Check sheet for the drawn part. Datum: minimum x, y, z corner. Units: mm. Give positions to 0.01 mm unless a question says otherwise; leave off trailing zeros. Order: outer loops, then holes, each group sorted by start corner. A loop starts at its lowest first (then second) coordinate and runs counter-clockwise, first axis right, second up.
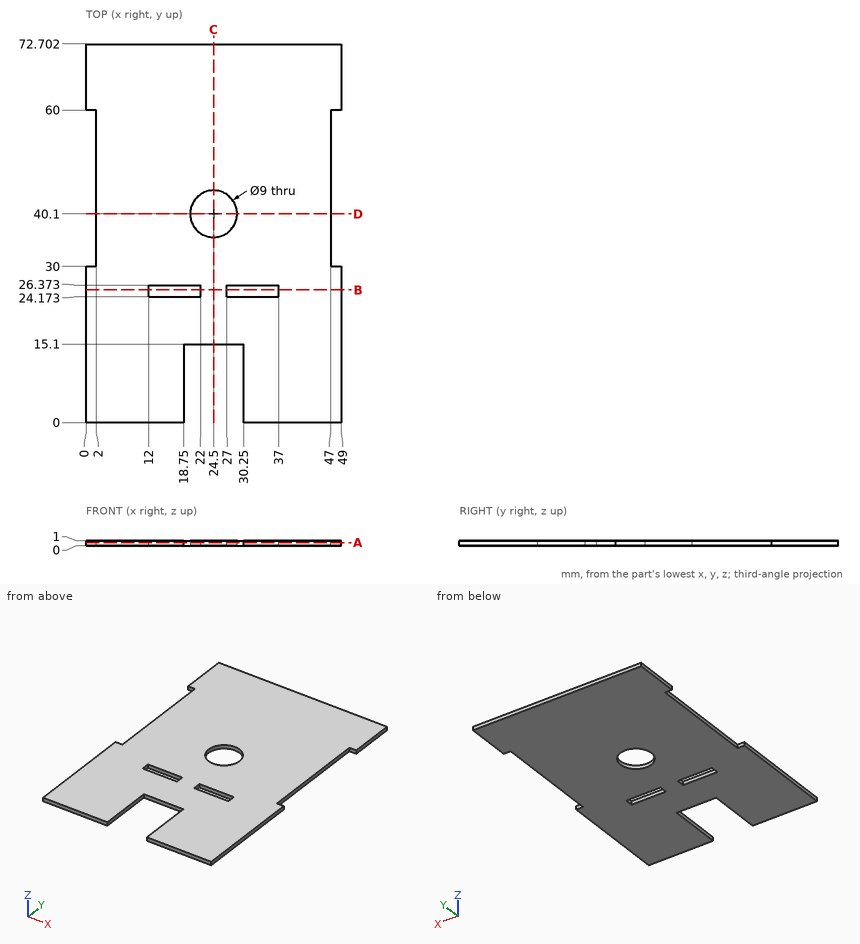
(1) Section check A-A, the plane z = 0.65. Enter the section's corners in (x, y).
Solved:
outline: (0, 0) - (18.75, 0) - (18.75, 15.1) - (30.25, 15.1) - (30.25, 0) - (49, 0) - (49, 30) - (47, 30) - (47, 60) - (49, 60) - (49, 72.7) - (0, 72.7) - (0, 60) - (2, 60) - (2, 30) - (0, 30) - close; hole (12, 24.17) - (22, 24.17) - (22, 26.37) - (12, 26.37) - close; hole circle Ø9 at (24.5, 40.1); hole (27, 24.17) - (37, 24.17) - (37, 26.37) - (27, 26.37) - close
(2) Go/stop test with flat-tipped pins: pin 1 (0.5 mm diameter, centred on x = 22, z = 0.5, fed in from -Y); pin 2 (0.5 mm diameter, centred on y = 46, z = 0.5, fed in from -X); pin 3 (8 mm diameter, centred on x = 24.5, y = 40.1, fed in from +Z). Record where each tip stops, or that it passes through.
Solved:
pin 1: stops at y = 15.1
pin 2: stops at x = 2
pin 3: passes through
(3) Scan lines: line 1 (Y direction, x = 24.5, z = 0.6); line 2 (X direction, y = 24.5, z = 0.8); line 3 (Y direction, x = 16.5, z = 0.8). Record each from-to range of solid material in increasing order.
Solved:
line 1: y = 15.1 to 35.6, 44.6 to 72.7
line 2: x = 0 to 12, 22 to 27, 37 to 49
line 3: y = 0 to 24.17, 26.37 to 72.7
(4) Section check B-B, the plane y = 25.5. Enter the section's corners in (x, z), then the cut area to 3 significant figures.
Solved:
outline: (0, 0) - (12, 0) - (12, 1) - (0, 1) - close; (22, 0) - (27, 0) - (27, 1) - (22, 1) - close; (37, 0) - (49, 0) - (49, 1) - (37, 1) - close
area: 29.0 mm2
(5) Section check D-D, the plane y = 40.1. Enter the section's corners in (x, z).
Solved:
outline: (2, 0) - (20, 0) - (20, 1) - (2, 1) - close; (29, 0) - (47, 0) - (47, 1) - (29, 1) - close
(6) Section check C-C, the plane x = 24.5. Enter the section's corners in (y, z).
Solved:
outline: (15.1, 0) - (35.6, 0) - (35.6, 1) - (15.1, 1) - close; (44.6, 0) - (72.7, 0) - (72.7, 1) - (44.6, 1) - close
